from build123d import *

# Parameters (mm, degrees)
F0_W         = 200
F0_H         = 30
F1_DEPTH     = 60
F2_SIZE      = 55
F3_SIZE      = 55
F4_W         = 54
F4_H         = 30
F5_DEPTH     = 55
F7_DEPTH     = 15
F8_R         = 10
F9_R         = 4.99999
F11_DEPTH    = 15
F12_T4_DEPTH = 73
F12_T9_DEPTH = 73
F13_R        = 10


# Not quite as in the source:
# - a fillet or chamfer that OpenCascade refuses, or shapes differently, is made with other operations: its cross-section is extruded or revolved along the edge and cut away or added
# - a fillet or chamfer is up to 0.001 mm smaller than in the source, because OpenCascade refuses the exact size


with BuildPart() as f1:
    # F0 (on Top) → F1 (new body)
    with BuildSketch(Plane.XY):
        with Locations((75.0721136101, 7.3799993843)):
            Rectangle(F0_W, F0_H)
    extrude(amount=F1_DEPTH)

    # F2
    f2_edges = [f1.edges().sort_by_distance(p)[0] for p in [
        (175.072114, 7.379999, 60),
    ]]
    chamfer(f2_edges, length=F2_SIZE)

    # F3
    f3_edges = [f1.edges().sort_by_distance(p)[0] for p in [
        (-24.927886, 7.379999, 60),
    ]]
    chamfer(f3_edges, length=F3_SIZE)

    # F4 (on face) → F5 (cut)
    with BuildSketch(Plane.XY.offset(60)):
        with Locations((75.0721136101, 7.3799993843)):
            Rectangle(F4_W, F4_H)
    extrude(amount=-F5_DEPTH, mode=Mode.SUBTRACT)

    # F6 (on face) → F7 (join)
    with BuildSketch(Plane.XZ.offset(7.6200006157)):
        Polygon((48.0721136101, 5), (-24.9278863899, 5), (-24.9278863899, 0), (175.0721136101, 0), (175.0721136101, 5), (102.0721136101, 5), align=None)
    extrude(amount=F7_DEPTH)

    # F8
    f8_edges = [f1.edges().sort_by_distance(p)[0] for p in [
        (175.072114, -22.620001, 2.5),
        (-24.927886, -22.620001, 2.5),
    ]]
    fillet(f8_edges, radius=F8_R)

    # F9 (radius 5 in the source; OpenCascade refuses exactly that, so slightly less here)
    f9_edges = [f1.edges().sort_by_distance(p)[0] for p in [
        (138.572114, -7.620001, 5),
        (11.572114, -7.620001, 5),
    ]]
    fillet(f9_edges, radius=F9_R)

    # F10 (on face) → F11 (join)
    with BuildSketch(Plane(origin=(0, 22.3799993843, 0), x_dir=(-1, 0, 0), z_dir=(0, 1, 0))):
        Polygon((-102.0721136101, 5), (-175.0721136101, 5), (-175.0721136101, 0), (24.9278863899, 0), (24.9278863899, 5), (-48.0721136101, 5), align=None)
    extrude(amount=F11_DEPTH)

    # F12: fillet of radius 5 on 2 edges, made by hand


with BuildPart() as f12_tool2:
    # F12_s3 → F12_t4 (new body)
    with BuildSketch(Plane.YZ.offset(102.0721136101)):
        with BuildLine():
            ThreePointArc((27.3799993843, 5), (23.8444654784, 6.4644660941), (22.3799993843, 10))
            Line((22.3799993843, 10), (22.3799993843, 5))
            Line((22.3799993843, 5), (27.3799993843, 5))
        make_face()
    extrude(amount=F12_T4_DEPTH)

    split(bisect_by=Plane(origin=(90.0360568051, 0, 90.0360568051), x_dir=(0, 1, 0), z_dir=(-0.7071067812, 0, -0.7071067812)), keep=Keep.TOP)


with BuildPart() as f1_1:
    add(f1.part)

    # F12_t1: union F12_tool2
    add(f12_tool2.part)


with BuildPart() as f12_tool7:
    # F12_s8 → F12_t9 (new body)
    with BuildSketch(Plane.YZ.offset(-24.9278863899)):
        with BuildLine():
            ThreePointArc((27.3799993843, 5), (23.8444654784, 6.4644660941), (22.3799993843, 10))
            Line((22.3799993843, 10), (22.3799993843, 5))
            Line((22.3799993843, 5), (27.3799993843, 5))
        make_face()
    extrude(amount=F12_T9_DEPTH)

    split(bisect_by=Plane(origin=(-14.9639431949, 0, 14.9639431949), x_dir=(0, 1, 0), z_dir=(0.7071067812, 0, -0.7071067812)), keep=Keep.TOP)


with BuildPart() as f1_2:
    add(f1_1.part)

    # F12_t6: union F12_tool7
    add(f12_tool7.part)

    # F13
    f13_edges = [f1_2.edges().sort_by_distance(p)[0] for p in [
        (175.072114, 37.379999, 2.5),
        (-24.927886, 37.379999, 2.5),
        (120.072114, 7.379999, 60),
        (30.072114, 7.379999, 60),
    ]]
    fillet(f13_edges, radius=F13_R)


solid = f1_2.part
Geometry: final body of the model. Coordinates: model frame, mm. A direction names the side the tool comes from. Round coordinates to 2 decimals unless told otherwise and drop trailing zeros. Write each loop counter-clockwise with the first axis right and the second up, starting at its lowest first coordinate (ties: lowest second). Pieces come first, ordered by that corner, then holes. Notation, with made-up numbers: M -11,-12 L 24,-12 A22 ccw 24,-5 Z; hole C 76,13 d11. An arc over 180 degrees is marked long. Write item = value, one per line.
Item 1: Section query A-A on z = 15. Return loops of the section in (x, y), then the cut area to 3 significant figures.
Findings:
outline = M -14.93,-7.62 L 48.07,-7.62 L 48.07,22.38 L -14.93,22.38 Z; M 102.07,-7.62 L 165.07,-7.62 L 165.07,22.38 L 102.07,22.38 Z
area = 3,780 mm^2
Item 2: Section query D-D on z = 53.5. Return loops of the section in (x, y), then the cut area to 3 significant figures.
Findings:
outline = M 23.57,-7.62 L 48.07,-7.62 L 48.07,22.38 L 23.57,22.38 Z; M 102.07,-7.62 L 126.57,-7.62 L 126.57,22.38 L 102.07,22.38 Z
area = 1,470 mm^2
Item 3: Section query C-C on x = 39.5. Return loops of the section in (y, z).
Findings:
outline = M -22.62,0 L 37.38,0 L 37.38,5 L 27.38,5 A5 cw 22.38,10 L 22.38,60 L -7.62,60 L -7.62,10 A5 cw -12.62,5 L -22.62,5 Z
Item 4: Access query for faces 1 (the face through (21, -7.62, 29)), 2 (the face through (149.4, 7.1, 30.67)). Directions: +Z, -Z, +X, -X, +Y, -Y. A direction counts if a zero-diameter tool reaches every point of the face in a straight line with its end or side. Return the directions, or none.
Findings:
face_1 = +Z, +X, -X, -Y
face_2 = +Z, +X, +Y, -Y
Item 5: Section query B-B on y = 6.5. Return loops of the section in (x, z).
Findings:
outline = M -24.93,0 L 175.07,0 L 175.07,5 L 123,57.07 A10 ccw 115.93,60 L 102.07,60 L 102.07,5 L 48.07,5 L 48.07,60 L 34.21,60 A10 ccw 27.14,57.07 L -24.93,5 Z
Item 6: Pin query (flat end, axial travel): P1, Ø8, axis at x = 16, z = 27.5, coming from the +Y side; P2, Ø2, axis at y = 6.5, z = 29, coming from the +X side; P3, Ø2, axis at x = 132, z = 24, coming from the -Y side. Return the tip coordinate at first contact, or that it passes through.
Findings:
P1 = 22.38
P2 = 152.07
P3 = -7.62
Item 7: Material intervals for line 1 along Y through (x, z) = (48, 10.5); line 2 along X through (y, z) = (16, 50.5); line 3 along X through (y, z) = (1, 40.5), sorted ascending. Write a range as [from, to].
Findings:
line_1 = [-7.62, 22.38]
line_2 = [20.57, 48.07], [102.07, 129.57]
line_3 = [10.57, 48.07], [102.07, 139.57]
Item 8: Pull-direction query (X, two-part tool) for faces 3 (the face through (102.072, 7, 33)), 4 (the face through (175.072, 7, 3)), 5 (the face through (74, -22.62, 3)), 6 (the face through (48.072, 7, 33)); classes: pulls with the +X half, pulls with the -X half, needs draft (parallel to the pull), parting line crosses it, or undercut.
Findings:
face_3 = undercut
face_4 = pulls with the +X half
face_5 = needs draft
face_6 = undercut
